```python
from build123d import *

# Parameters (mm, degrees)
ESQUISSE1_W                  = 18
ESQUISSE1_H                  = 16
ESQUISSE1_R                  = 6
BASE_EXTRUSION_DEPTH         = 11.5
ESQUISSE6_R                  = 3.506411758
ENL_V_MAT_EXTRU_1_DEPTH      = 28.244265452
CHANFREIN1_SIZE              = 1
ESQUISSE9_W                  = 7.559075372
ESQUISSE9_H                  = 1.8
ENL_V_MAT_EXTRU_2_REACH      = 38.326
ENL_V_MAT_EXTRU_2_END_RADIUS = 1
ESQUISSE10_R                 = 1


with BuildPart() as part:
    # Esquisse1 → Base-Extrusion (new, symmetric)
    with BuildSketch(Plane.XY):
        with Locations((0, 8)):
            Rectangle(ESQUISSE1_W, ESQUISSE1_H)
        with Locations((0, 8)):
            Circle(ESQUISSE1_R, mode=Mode.SUBTRACT)
    extrude(amount=BASE_EXTRUSION_DEPTH, both=True)

    # Esquisse5 → Boss.-Révol.1 (revolve)
    with BuildSketch(Plane(origin=(0, 0, 0), x_dir=(0, 0, -1), z_dir=(1, 0, 0)), mode=Mode.PRIVATE) as boss_r_vol_1_sk:
        Polygon((7, -10), (7, -11), (5.5, -11), (3.506411758, 0), (7, 0), (7, -8.8), (5.8, -8.8), (5.8, -10), align=None)
        Polygon((7, 16), (3.5, 16), (6, 23), (7, 23), align=None)
    revolve(boss_r_vol_1_sk.sketch.rotate(Axis((0, 26.536034952, 0), (0, -1, 0)), 180), axis=Axis((0, 26.536034952, 0), (0, -1, 0)))

    # Esquisse6 → Enlèv. mat.-Extru.1 (cut, through all)
    with BuildSketch(Plane.XZ):
        Circle(ESQUISSE6_R)
    extrude(amount=-ENL_V_MAT_EXTRU_1_DEPTH, mode=Mode.SUBTRACT)

    # Esquisse8 → Boss.-Révol.2 (revolve)
    with BuildSketch(Plane(origin=(0, 0, 0), x_dir=(0, 0, -1), z_dir=(1, 0, 0))):
        Polygon((-11.5, 15), (-16.5, 15), (-21.5, 13.180148829), (-21.5, 10), (-18.894611613, 10), (-18.894611613, 9), (-5.574935919, 9), (-5.574935919, 9.8), (-11.5, 9.8), align=None)
    revolve(axis=Axis((0, 8, 5.789251087), (0, 0, 1)))

    # Chanfrein1
    chanfrein1_edges = [part.edges().sort_by_distance(p)[0] for p in [
        (9, 16, 0),
        (9, 0, 0),
        (-9, 0, 0),
        (-9, 16, 0),
    ]]
    chamfer(chanfrein1_edges, length=CHANFREIN1_SIZE)

    # Esquisse9 → Boss.-Révol.3 (revolve)
    with BuildSketch(Plane(origin=(2.407260093, 7.19454204, 0), x_dir=(-0.9483236552062002, 0.31730465640508954, 0), z_dir=(0.31730465640508954, 0.9483236552062002, 0)), mode=Mode.PRIVATE) as boss_r_vol_3_sk:
        with Locations((10.758899565, 17.9)):
            Rectangle(ESQUISSE9_W, ESQUISSE9_H)
    revolve(boss_r_vol_3_sk.sketch.rotate(Axis((0, 8, 17), (-0.9483236552062002, 0.3173046564050896, 0)), 90), axis=Axis((0, 8, 17), (-0.9483236552062002, 0.3173046564050896, 0)))

    # Enlèv. mat.-Extru.2: up to this cylinder (the profile starts outside it)
    enl_v_mat_extru_2_end = Plane(origin=(0, 8, 17), z_dir=(0, 0, -1)) * Cylinder(ENL_V_MAT_EXTRU_2_END_RADIUS, 79.652, mode=Mode.PRIVATE)
    # Esquisse10 → Enlèv. mat.-Extru.2 (cut, up to the surface)
    with BuildSketch(Plane(origin=(-13.787143955, 4.613113837, 0), x_dir=(0, 0, 1), z_dir=(-0.9483236552062002, 0.31730465640508954, 0)), mode=Mode.PRIVATE) as enl_v_mat_extru_2_sk1:
        with Locations(Location((17, 7.586589242, 0), (0, 0, 270))):
            Circle(ESQUISSE10_R)
    enl_v_mat_extru_2_tool1 = extrude(enl_v_mat_extru_2_sk1.sketch, amount=-ENL_V_MAT_EXTRU_2_REACH, mode=Mode.PRIVATE) - enl_v_mat_extru_2_end
    add(enl_v_mat_extru_2_tool1.solids().sort_by_distance((-11.379884, 11.807656, 17))[0], mode=Mode.SUBTRACT)


solid = part.part
```
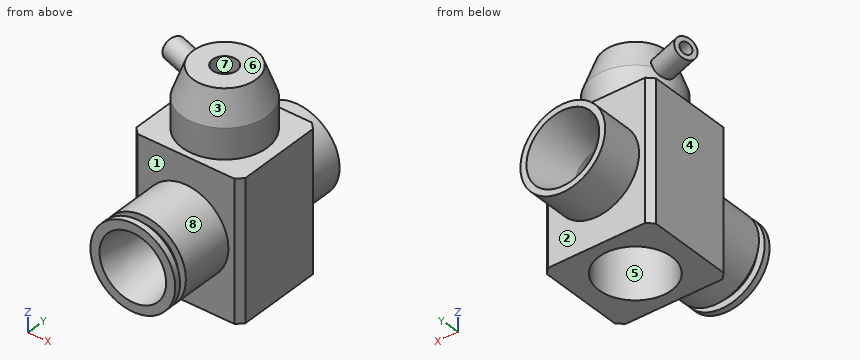
Verification items for the finished model (mm, model axes). Face numbers are marked on the shaded views. A direction names the side the tool comes from. Coordinates: 2 decimals unless noted, no trailing zeros. Order: outer loops, then holes, each group sorted by start corner. A loop starts at its lowest first (then second) coordinate and runs counter-clockwise, first axis right, second up. Notation, with made-up numbers: (68.25, -30) -> (119.25, -30) arc R5 cw to (119.25, -22) -> close; hole circle Ø7 at (47, -21.5). An arc over 180 degrees is marked (long way). Put each result on its own line as item: value. Start each with the question number.
1) Go/stop test with flat-tipped pins: pin 1 (3 mm diameter, centred on y = 16, z = 7, fed in from -X); pin 2 (8 mm diameter, centred on x = 1.5, y = 8, fed in from -Z); pin 3 (4 mm diameter, centred on y = -4.5, z = 1, fed in from +X); pin 4 (1.2 mm diameter, centred on x = 0, y = 8, fed in from +Z). Record where each tip stops, or that it passes through.
2) Release check for a two-part mould opening along X. For the marked faces 5, 6, 7 and 8 record: pulls with the +X half, pulls with the -X half, needs draft (parallel to the pull), parting line crosses it, or undercut.
3) Material ranges on L1, parallel to Y at x = 0, z = 9.5; L2, parallel to X at y = 13, z = 0; L3, parallel to X at y = -8, z = -1.5, recorded low to high.
4) Tool access check on the marked faces 1, 2, 3 and 4. Record the directions out of +Z, -Z, +X, -X, +Y, -Y that give a thin tool (end or side, any length) a straight path to the whole face; none if there is none.
5) Cross-section at B-B (y = -4). Enter the section's corners in (x, z), plus the area to 3 significant figures.
6) Cross-section at A-A (y = 20). Enter the section's corners in (x, z), plus the area to 3 significant figures.
Geometry check:
1. pin 1: stops at x = -9
1. pin 2: stops at z = 5.57
1. pin 3: stops at x = 7
1. pin 4: passes through
2. face 5: undercut
2. face 6: needs draft
2. face 7: undercut
2. face 8: parting line crosses it
3. L1: y = 0 to 2, 6.2 to 7, 9 to 9.8, 14 to 16
3. L2: x = -9 to -3.51, 3.51 to 9
3. L3: x = -6.84 to -4.72, 4.72 to 6.84
4. face 1: -Y
4. face 2: +Y
4. face 3: +Z
4. face 4: -Z, -X, +Y, -Y
5. outline: circle Ø14 at (0, 0); hole circle Ø8.46 at (0, 0)
5. area: 97.7 mm^2
6. outline: circle Ø14 at (0, 0); hole circle Ø9.86 at (0, 0)
6. area: 77.6 mm^2
